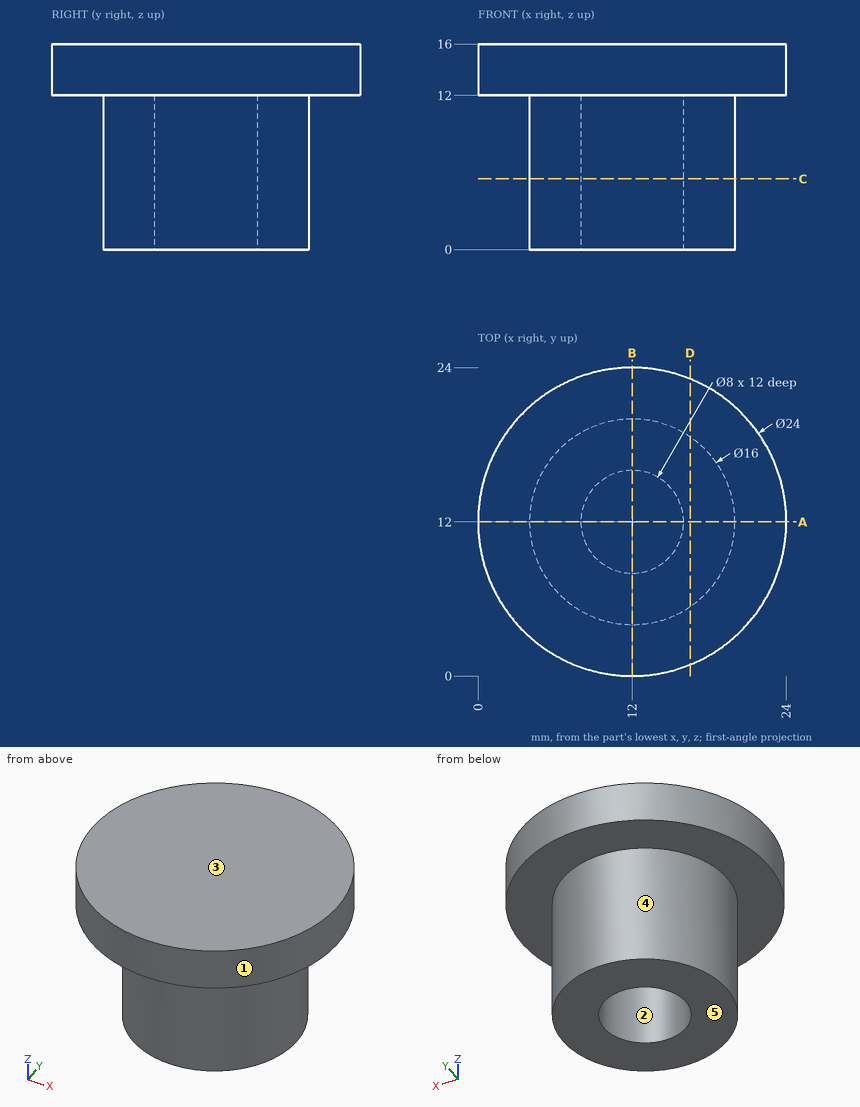
For this review, use the dimensioned drawing (mm, ordinates from the lowest corner) and the shaded views. A direction names the side the tool comes from. Round coordinates to 2 decimals unless told otherwise and drop trailing zeros. Write each loop counter-clockwise with the first axis right and the second up, starting at its lowest first coordinate (ties: lowest second). Pieces come first, ordered by that corner, then holes. Notation, with made-up numbers: (-2, -11.5) - (53, -11.5) arc R7 cw to (53, -7.5) - close; hole circle Ø3 at (-1, 26.5). An arc over 180 degrees is marked (long way). Use a Markdown table: item, result.
Q1. We need section D-D (x = 16.5). Give the boundary of the cut face in (y, z), plus the area to 3 significant figures.
Derived:
| item | result |
|---|---|
| outline | (0.88, 12) - (5.39, 12) - (5.39, 0) - (18.61, 0) - (18.61, 12) - (23.12, 12) - (23.12, 16) - (0.88, 16) - close |
| area | 248 mm2 |
Q2. We need section A-A (y = 12). Give the boundary of the cut face in (x, z), plus the area to 3 significant figures.
Derived:
| item | result |
|---|---|
| outline | (0, 12) - (4, 12) - (4, 0) - (8, 0) - (8, 12) - (16, 12) - (16, 0) - (20, 0) - (20, 12) - (24, 12) - (24, 16) - (0, 16) - close |
| area | 192 mm2 |
Q3. The part is to be moulded in two halves that separate along Y. For the marked faces 1, 2 and 3, say which applies: pulls with the +Y half, pulls with the -Y half, needs draft (parallel to the pull), parting line crosses it, or undercut.
Derived:
| item | result |
|---|---|
| face 1 | parting line crosses it |
| face 2 | undercut |
| face 3 | needs draft |
Q4. Wall thickness on line 1 along Y through (x, z) = (12, 4.75); line 2 along Z through (x, y) = (6, 4.5); line 3 along Y through (x, z) = (14.75, 2.25): over which ranges is each line inside the solid? List them lowest first.
Derived:
| item | result |
|---|---|
| line 1 | y = 4 to 8, 16 to 20 |
| line 2 | z = 12 to 16 |
| line 3 | y = 4.49 to 9.1, 14.9 to 19.51 |
Q5. Clearance check with flat-ended pins moving along their axes: pin 1 (8 mm diameter, centred on x = 16, z = 12.5, fed in from +Y); pin 2 (3 mm diameter, centred on y = 5, z = 9.5, fed in from -X); pin 3 (4 mm diameter, centred on x = 17, z = 3.5, fed in from -Y). State where each tip first meets the part, or that it passes through.
Derived:
| item | result |
|---|---|
| pin 1 | stops at y = 24 |
| pin 2 | stops at x = 6.19 |
| pin 3 | stops at y = 4.58 |
Q6. We need section C-C (z = 5.5). Give the boundary of the cut face in (x, y).
Derived:
| item | result |
|---|---|
| outline | circle Ø16 at (12, 12); hole circle Ø8 at (12, 12) |
Q7. Machinability: for the marked faces 4 and 5, which of the approach directions +Z, -Z, +X, -X, +Y, -Y give a long, thin tool a straight path to every point of the face, cutting with its end or side? Answer none if there is none.
Derived:
| item | result |
|---|---|
| face 4 | -Z |
| face 5 | -Z, +X, -X, +Y, -Y |
